Model file for the job. Use its own axes, mm. A direction names the side the tool comes from. Coordinates: 2 decimals unless noted, no trailing zeros. Write each loop counter-clockwise with the first axis right and the second up, starting at its lowest first coordinate (ties: lowest second). Pieces come first, ordered by that corner, then holes. Notation, with made-up numbers: M 14,-26 L 71,-26 A21 cw 71,-8 Z; hole C -26,-31.5 d10. An arc over 180 degrees is marked long. Use CSV: the item, a comma, the result in double quotes. Start each with the question number.
from build123d import *

# Parameters (mm, degrees)
F0_R     = 2.5
F1_DEPTH = 5
F2_W     = 0.1429862286
F2_H     = 0.6
F3_DEPTH = 25
F4_R     = 7
F5_DEPTH = 18
F6_R     = 5.5
F7_DEPTH = 4
F8_R     = 7
F9_DEPTH = 7


with BuildPart() as f1:
    # F0 (on Front) → F1 (new body)
    with BuildSketch(Plane.XZ):
        Circle(F0_R)
    extrude(amount=F1_DEPTH)

    # F2 (on face) → F3 (cut)
    with BuildSketch(Plane.XZ.offset(5)):
        with Locations((-2.5534278435, 0)):
            Rectangle(F2_W, F2_H)
    extrude(amount=-F3_DEPTH, mode=Mode.SUBTRACT)

    # F4 (on face) → F5 (join)
    with BuildSketch(Plane(origin=(-2.4819347292, 0, 0), x_dir=(0, -1, 0), z_dir=(-1, 0, 0))):
        with Locations((-3.8429031865, 0)):
            Circle(F4_R)
    extrude(amount=-F5_DEPTH)

    # F6 (on face) → F7 (join)
    with BuildSketch(Plane(origin=(-2.4819347292, 0, 0), x_dir=(0, -1, 0), z_dir=(-1, 0, 0))):
        with Locations((-3.8429031865, 0)):
            Circle(F6_R)
    extrude(amount=F7_DEPTH)

    # F8 (on face) → F9 (join)
    with BuildSketch(Plane(origin=(-6.4819347292, 0, 0), x_dir=(0, -1, 0), z_dir=(-1, 0, 0))):
        with Locations((-3.8429031865, 0)):
            Circle(F8_R)
    extrude(amount=F9_DEPTH)


solid = f1.part
1) Band-saw the part on A-A on z = 0. List the corners of the cut face in (x, y).
2) Band-saw the part on D-D on x = 0. List the corners of the cut face in (y, z).
3) Drop flat-ended pins along their axis: P1, Ø4, axis at x = -3.5, y = 2, coming from the -Z side; P2, Ø2, axis at x = 4.5, z = 0.5, coming from the -Y side; P3, Ø2, axis at x = 11, z = -1.5, coming from the +Y side (3 decimals). Give the stop position or say it passes through.
4) Tool access for faces 1 (the face through (-2.482, -2, 0)), 2 (the face through (15.518, 4, 0)), 3 (the face through (2.5, -3.8, -0.1)): list every direction of +Z, -Z, +X, -X, +Y, -Y with a clear straight run to the whole face (end or side of a thin tool).
5) Band-saw the part on B-B on y = -2. List the corners of the cut face in (x, z), then the cut area to 3 significant figures.
6) Band-saw the part on C-C on y = 7.5. List the corners of the cut face in (x, z), then the cut area to 3 significant figures.
7) Wall check: L1, parallel to X at y = 4.25, z = 6.5; L2, parallel to Z at x = -4, y = 3.75; L3, parallel to Z at x = -5.5, y = 2.75. Give the ranges that are in metal, low to high. Write a range as [from, to].
8) Two-plate mould, pull along X, no slides. Class faces 4 (the face through (0, -5, 0)), 5 (the face through (-4.454, 9.338, 0.242)), 6 (the face through (-13.482, 4, 0)): pulls with the +X half, pulls with the -X half, needs draft (parallel to the pull), parting line crosses it, or undercut.
Findings below:
1,outline,"M -13.48,-3.16 L -6.48,-3.16 L -6.48,-1.66 L -2.48,-1.66 L -2.48,-5 L 2.5,-5 L 2.5,-3.16 L 15.52,-3.16 L 15.52,10.84 L -2.48,10.84 L -2.48,9.34 L -6.48,9.34 L -6.48,10.84 L -13.48,10.84 Z"
2,outline,"M -5,-2.5 L -2.7,-2.5 A7 ccw long -2.7,2.5 L -5,2.5 Z"
3,P1,"stops at z = -7"
3,P2,"stops at y = -3.16"
3,P3,"stops at y = 10.825"
4,face 1,"none"
4,face 2,"+Z, -Z, +X, +Y, -Y"
4,face 3,"-Y"
5,outline,"M -13.48,-3.85 L -6.48,-3.85 L -6.48,3.85 L -13.48,3.85 Z; M -2.48,-3.85 L 15.52,-3.85 L 15.52,3.85 L -2.48,3.85 Z"
5,area,"193 mm2"
6,outline,"M -13.48,-5.97 L -6.48,-5.97 L -6.48,-4.11 L -2.48,-4.11 L -2.48,-5.97 L 15.52,-5.97 L 15.52,5.97 L -2.48,5.97 L -2.48,4.11 L -6.48,4.11 L -6.48,5.97 L -13.48,5.97 Z"
6,area,"331 mm2"
7,L1,"x = [-13.48, -6.48], [-2.48, 15.52]"
7,L2,"z = [-5.5, 5.5]"
7,L3,"z = [-5.39, 5.39]"
8,face 4,"needs draft"
8,face 5,"undercut"
8,face 6,"pulls with the -X half"
